```python
from build123d import *

# Parameters (mm, degrees)
SKETCH_1_R                   = 46
EXTRUDE_1_DEPTH              = 31.6
SKETCH_2_R                   = 41.5
EXTRUDE_2_DEPTH              = 13
SKETCH_3_R                   = 26.5
EXTRUDE_3_DEPTH              = 13.5
SKETCH_4_R                   = 1.5
CUT_EXTRUDE_1_DEPTH          = 10
HOLE_WIZARD_M4_1_D           = 3.3
HOLE_WIZARD_M4_1_DEPTH       = 10.1
HOLE_WIZARD_M4_1_TIP         = 0.991420021
HOLE_WIZARD_M3_1_D           = 3.4
HOLE_WIZARD_M3_1_DEPTH       = 7.5
HOLE_WIZARD_M3_1_CBORE_D     = 6
HOLE_WIZARD_M3_1_CBORE_DEPTH = 3.4
HOLE_WIZARD_M3_1_TIP         = 1.021463052
SKETCH_9_W                   = 30
SKETCH_9_H                   = 15
EXTRUDE_4_DEPTH              = 4


with BuildPart() as part:
    # 草图1 → 凸台-拉伸1 (new body)
    with BuildSketch(Plane(origin=(0, 0, 0), x_dir=(1, 0, 0), z_dir=(0, 1, 0))):
        Circle(SKETCH_1_R)
    extrude(amount=EXTRUDE_1_DEPTH)

    # 草图2 → 凸台-拉伸2 (add)
    with BuildSketch(Plane(origin=(0, 31.6, 0), x_dir=(1, 0, 0), z_dir=(0, 1, 0))):
        Circle(SKETCH_2_R)
    extrude(amount=EXTRUDE_2_DEPTH)

    # 草图3 → 凸台-拉伸3 (add)
    with BuildSketch(Plane(origin=(0, 31.6, 0), x_dir=(1, 0, 0), z_dir=(0, 1, 0))):
        Circle(SKETCH_3_R)
    extrude(amount=EXTRUDE_3_DEPTH)

    # 草图4 → 切除-拉伸1 (cut)
    with BuildSketch(Plane(origin=(0, 45.1, 0), x_dir=(1, 0, 0), z_dir=(0, 1, 0))):
        with Locations((-21.75, 0)):
            Circle(SKETCH_4_R)
        with Locations((21.75, 0)):
            Circle(SKETCH_4_R)
        with Locations((13.980630511, 16.661466638)):
            Circle(SKETCH_4_R)
        with Locations((-13.980630511, 16.661466638)):
            Circle(SKETCH_4_R)
        with Locations((13.980630511, -16.661466638)):
            Circle(SKETCH_4_R)
        with Locations((-13.980630511, -16.661466638)):
            Circle(SKETCH_4_R)
    extrude(amount=-CUT_EXTRUDE_1_DEPTH, mode=Mode.SUBTRACT)

    # M4 螺纹孔1
    with Locations(Plane(origin=(-13.980630511, 45.1, 16.661466638), x_dir=(0, 0, 1), z_dir=(0, 1, 0))):
        with Locations((0, 0), (-16.661466638, -7.769369489), (-33.322933276, 0), (-33.322933276, 27.961261022), (-16.661466638, 35.730630511), (0, 27.961261022)):
            Hole(HOLE_WIZARD_M4_1_D / 2, depth=HOLE_WIZARD_M4_1_DEPTH)
            with Locations((0, 0, -(HOLE_WIZARD_M4_1_DEPTH + HOLE_WIZARD_M4_1_TIP / 2))):  # 118° drill point
                Cone(0, HOLE_WIZARD_M4_1_D / 2, HOLE_WIZARD_M4_1_TIP, mode=Mode.SUBTRACT)

    # M3 六角圆柱头螺钉的柱形沉头孔1
    with Locations(Plane(origin=(32.04293994, 44.6, -18.5), x_dir=(0, 0, 1), z_dir=(0, 1, 0))):
        with Locations((0, 0), (37, 0), (55.5, -32.04293994), (37, -64.08587988), (0, -64.08587988), (-18.5, -32.04293994)):
            CounterBoreHole(HOLE_WIZARD_M3_1_D / 2, HOLE_WIZARD_M3_1_CBORE_D / 2, HOLE_WIZARD_M3_1_CBORE_DEPTH, depth=HOLE_WIZARD_M3_1_DEPTH)
            with Locations((0, 0, -(HOLE_WIZARD_M3_1_DEPTH + HOLE_WIZARD_M3_1_TIP / 2))):  # 118° drill point
                Cone(0, HOLE_WIZARD_M3_1_D / 2, HOLE_WIZARD_M3_1_TIP, mode=Mode.SUBTRACT)

    # 草图9 → 凸台-拉伸4 (add)
    with BuildSketch(Plane.XZ):
        with Locations((1.722788181, -26.5)):
            Rectangle(SKETCH_9_W, SKETCH_9_H)
    extrude(amount=EXTRUDE_4_DEPTH)


solid = part.part
```
Can you work these out from the model? Positions are in its coordinate system, mm. A direction names the side the tool comes from. Coordinates: 2 decimals unless noted, no trailing zeros. Write each loop counter-clockwise with the first axis right and the second up, starting at its lowest first coordinate (ties: lowest second). Pieces come first, ordered by that corner, then holes. Notation, with made-up numbers: M -38.5,21 L -9.5,21 A32 ccw -9.5,54 Z; hole C 15,79.25 d10. An arc over 180 degrees is marked long. Write item = value, one per line. Start each with the question number.
Q1. If we section it at A-A, the plane y = 39: State how many separate pieces and enclosed holes the cut face has, then the cut area to 3 significant figures.
Q2. If we section it at D-D, the plane y = 3.5: Write out the boundary of the cut face in (x, z).
Q3. I'm going to push flat-ended pins straight in: pin 1 (3 mm diameter, centred on x = -17.5, z = 32, fed in from +Y); pin 2 (1.5 mm diameter, centred on y = 15, z = -28, fed in from -X); pin 3 (3 mm diameter, centred on x = -32.04, z = -18.5, fed in from +Y). Where does each tip first touch, or does it pass through?
Q4. On a 3-axis mill with a long thin cutter (end or side, diameter ignored), from which of +Z, -Z, +X, -X, +Y, -Y can I reach the whole of each face in a straight line? I mean faces 1 (the face through (2, -2, -19)), 2 (the face through (0, 41.2, -35)), 3 (the face through (2, -4, -26)). Say none if no direction works.
Q5. If I drill on L1, parallel to X at y = 38, z = 0; L2, parallel to X at y = 43.8, z = -18.5; L3, parallel to Y at x = 33.5, z = 14, over which ranges is the centre line in solid material (lowest first)? Write a range as [from, to].
Q6. If we section it at B-B, the plane x = -5: Write out the boundary of the cut face in (y, z), then the cut area to 3 significant figures.
Q7. Thinking about a two-plate mould opening in X: for faces 4 (the face through (22.03, 34.18, -0.04)), 5 (the face through (-1, 44.6, 27)), 6 (the face through (-5.99, 15.58, -45.61)), which applies, released by +X, released by -X, zero draft, split by the parting line, or undercut?
Q8. If we section it at C-C, the plane z = -5: Write out the boundary of the cut face in (x, y), then the cut area to 3 significant figures.
Check sheet entries:
q1.separate_pieces = 1
q1.enclosed_holes = 12
q1.area = 5,300 mm²
q2.outline = C 0,0 d92
q3.pin_1 = 44.6
q3.pin_2 = -37.06
q3.pin_3 = 36.98
q4.face_1 = +Z, +X, -X, -Y
q4.face_2 = +Y
q4.face_3 = +Z, -Z, +X, -X, -Y
q5.L1 = [-41.5, -23.4], [-20.1, 20.1], [23.4, 41.5]
q5.L2 = [-37.15, -35.04], [-29.04, 29.04], [35.04, 37.15]
q5.L3 = [0, 44.6]
q6.outline = M -4,-34 L 0,-34 L 0,-45.73 L 31.6,-45.73 L 31.6,-41.2 L 44.6,-41.2 L 44.6,-26.02 L 45.1,-26.02 L 45.1,26.02 L 44.6,26.02 L 44.6,41.2 L 31.6,41.2 L 31.6,45.73 L 0,45.73 L 0,-19 L -4,-19 Z
q6.area = 4,050 mm²
q7.face_4 = undercut
q7.face_5 = zero draft
q7.face_6 = split by the parting line
q8.outline = M -45.73,0 L 45.73,0 L 45.73,31.6 L 41.2,31.6 L 41.2,44.6 L 26.02,44.6 L 26.02,45.1 L -26.02,45.1 L -26.02,44.6 L -41.2,44.6 L -41.2,31.6 L -45.73,31.6 Z
q8.area = 3,990 mm²
